Could you check a few things on this model? Use its own coordinates, in mm. A direction names the side the tool comes from. Coordinates: 2 decimals unless noted, no trailing zeros. Order: outer loops, then holes, each group sorted by start corner. A loop starts at its lowest first (then second) coordinate and runs counter-clockwise, first axis right, second up. Notation, with made-up numbers: (58, 51) - (77, 51) arc R13 cw to (77, 57) - close; hole circle Ø1 at (3, -14). An arc over 180 degrees is marked (long way). Answer as a JSON object with one key per item and string values. Group by question number.
(1) Imagine slicing it at D-D, the plane z = 5.25. Give the number of separate pieces and of enclosed holes in the cut face, and give its area (3 significant figures).
(2) Will this pin go through, and if not, where does the flat tip stop? P1, Ø0.5, axis at y = -43.5, z = 6.5, coming from the -X side.
(3) Please list where these lines run through material, in increasing order: probe 1 along Y at (x, z) = (-43.8, 2.75); probe 2 along Y at (x, z) = (-7, 4.5); probe 3 along Y at (x, z) = (43.8, 3.5).
(4) Imagine slicing it at C-C, the plane y = 24.4. Write out the boundary of the cut face in (x, z).
(5) Imagine slicing it at A-A, the plane x = -21.5. Write out the boundary of the cut face in (y, z), and give its area (3 significant figures).
(6) We'd pull the mould along X, two halves only. Please class faces 1 (the flat face through (54.3, 30, 3)), 2 (the cylindrical face through (-52.96, 46.287, 3.296)), 3 (the cylindrical face through (48.33, -43.97, 1.01)), 4 (the cylindrical face through (-48.12, 42.39, 4.75)): pulls with the +X half, pulls with the -X half, needs draft (parallel to the pull), parting line crosses it, or undercut.
(7) Imagine slicing it at B-B, the plane x = -43.8. Write out the boundary of the cut face in (y, z), and give its area (3 significant figures).
(8) Which directions (+Z, -Z, +X, -X, +Y, -Y) give clear straight access to the entire face, cutting with the end or side of a thin tool? Please do faces 5 (the cylindrical face through (-48.12, -43.61, 1.01)), 6 (the cylindrical face through (51.91, 11.77, 3.3)), 7 (the cylindrical face through (50.352, -26.595, 7.955)).
from build123d import *

# Parameters (mm, degrees)
SKETCH1_W                = 108.6
SKETCH1_H                = 95.4
BOSS_EXTRUDE1_DEPTH      = 6.5
FILLET1_R                = 4.7
CUT_EXTRUDE2_DEPTH       = 73.567416931
SHELL1_T                 = -3
SHELL1_THICKNESS_2_DEPTH = 1
SKETCH3_W                = 21
SKETCH3_H                = 9.8
CUT_EXTRUDE1_DEPTH       = 73.567416931
BOSS_EXTRUDE2_START      = 2.87
BOSS_EXTRUDE2_DEPTH      = 2.87
SKETCH6_R                = 1.6
CUT_EXTRUDE3_DEPTH       = 73.650512042
BOSS_EXTRUDE3_START      = 7.37
SKETCH7_R                = 4.5
SKETCH7_R_2              = 1.6
BOSS_EXTRUDE3_DEPTH      = 7.37


with BuildPart() as part:
    # Sketch1 → Boss-Extrude1 (new body)
    with BuildSketch(Plane.XY):
        Rectangle(SKETCH1_W, SKETCH1_H)
    extrude(amount=BOSS_EXTRUDE1_DEPTH)

    # Fillet1
    fillet1_edges = [part.edges().sort_by_distance(p)[0] for p in [
        (54.3, -47.7, 3.25),
        (-54.3, -47.7, 3.25),
        (-54.3, 47.7, 3.25),
        (54.3, 47.7, 3.25),
    ]]
    fillet(fillet1_edges, radius=FILLET1_R)

    # Sketch4 → Cut-Extrude2 (cut, through all)
    with BuildSketch(Plane.XY.offset(6.5)):
        with BuildLine():
            Line((50.037, 6.46747704), (50.037, -20.87017704))
            ThreePointArc((50.037, -20.87017704), (146.29602, -7.20135), (50.037, 6.46747704))
        make_face()
    extrude(amount=-CUT_EXTRUDE2_DEPTH, mode=Mode.SUBTRACT)

    # Shell1
    shell1_openings = [part.faces().sort_by_distance(p)[0] for p in [
        (-0.847501067, 0.116576538, 6.5),
    ]]
    offset(amount=SHELL1_T, openings=shell1_openings, kind=Kind.INTERSECTION)

    # Shell1 thickness 2 face (on inner face of the shell) → Shell1 thickness 2 (cut)
    with BuildSketch(Plane(origin=(-0.931808726, 0.135963236, 3), x_dir=(-1, 0, 0), z_dir=(0, 0, -1))):
        with BuildLine():
            ThreePointArc((50.368191274, -43.135963236), (49.870272802, -44.338044764), (48.668191274, -44.835963236))
            Line((48.668191274, -44.835963236), (-50.531808726, -44.835963236))
            ThreePointArc((-50.531808726, -44.835963236), (-51.733890254, -44.338044764), (-52.231808726, -43.135963236))
            Line((-52.231808726, -43.135963236), (-52.231808726, -31.994266579))
            ThreePointArc((-52.231808726, -31.994266579), (-49.810478696, -26.826892146), (-47.968808726, -21.425702521))
            Line((-47.968808726, -21.425702521), (-47.968808726, 6.751076049))
            ThreePointArc((-47.968808726, 6.751076049), (-49.810478696, 12.152265674), (-52.231808726, 17.319640107))
            Line((-52.231808726, 17.319640107), (-52.231808726, 42.864036764))
            ThreePointArc((-52.231808726, 42.864036764), (-51.733890254, 44.066118292), (-50.531808726, 44.564036764))
            Line((-50.531808726, 44.564036764), (48.668191274, 44.564036764))
            ThreePointArc((48.668191274, 44.564036764), (49.870272802, 44.066118292), (50.368191274, 42.864036764))
            Line((50.368191274, 42.864036764), (50.368191274, -43.135963236))
        make_face()
    extrude(amount=SHELL1_THICKNESS_2_DEPTH, mode=Mode.SUBTRACT)

    # Sketch3 → Cut-Extrude1 (cut, through all)
    with BuildSketch(Plane.XY.offset(6.5)):
        with Locations((-15.1, -31.9)):
            Rectangle(SKETCH3_W, SKETCH3_H)
        with Locations((15.3, -31.9)):
            Rectangle(SKETCH3_W, SKETCH3_H)
    extrude(amount=-CUT_EXTRUDE1_DEPTH, mode=Mode.SUBTRACT)

    # Sketch5 → Boss-Extrude2 (add)
    with BuildSketch(Plane.XY.offset(6.5).offset(BOSS_EXTRUDE2_START)):
        with BuildLine():
            Line((52.7, 17.100794024), (52.7, 43))
            ThreePointArc((52.7, 43), (51.792031022, 45.192031022), (49.6, 46.1))
            Line((49.6, 46.1), (-49.6, 46.1))
            ThreePointArc((-49.6, 46.1), (-51.792031022, 45.192031022), (-52.7, 43))
            Line((-52.7, 43), (-52.7, -43))
            ThreePointArc((-52.7, -43), (-51.792031022, -45.192031022), (-49.6, -46.1))
            Line((-49.6, -46.1), (49.6, -46.1))
            ThreePointArc((49.6, -46.1), (51.792031022, -45.192031022), (52.7, -43))
            Line((52.7, -43), (52.7, -31.503494024))
            ThreePointArc((52.7, -31.503494024), (50.322512039, -26.523985726), (48.500249857, -21.315597065))
            Line((48.500249857, -21.315597065), (47.044269983, -21.315597065))
            ThreePointArc((47.044269983, -21.315597065), (48.883695535, -26.70338335), (51.3, -31.858303343))
            Line((51.3, -31.858303343), (51.3, -43))
            ThreePointArc((51.3, -43), (50.802081528, -44.202081528), (49.6, -44.7))
            Line((49.6, -44.7), (-49.6, -44.7))
            ThreePointArc((-49.6, -44.7), (-50.802081528, -44.202081528), (-51.3, -43))
            Line((-51.3, -43), (-51.3, 43))
            ThreePointArc((-51.3, 43), (-50.802081528, 44.202081528), (-49.6, 44.7))
            Line((-49.6, 44.7), (49.6, 44.7))
            ThreePointArc((49.6, 44.7), (50.802081528, 44.202081528), (51.3, 43))
            Line((51.3, 43), (51.3, 17.455603343))
            ThreePointArc((51.3, 17.455603343), (48.883695535, 12.30068335), (47.044269983, 6.912897065))
            Line((47.044269983, 6.912897065), (48.500249857, 6.912897065))
            ThreePointArc((48.500249857, 6.912897065), (50.322512039, 12.121285726), (52.7, 17.100794024))
        make_face()
    extrude(amount=-BOSS_EXTRUDE2_DEPTH)

    # Sketch6 → Cut-Extrude3 (cut, through all)
    with BuildSketch(Plane.XY.offset(2)):
        with Locations((-49.6, 43)):
            Circle(SKETCH6_R)
        with Locations((-43.8, 24.4)):
            Circle(SKETCH6_R)
        with Locations((43.8, 24.4)):
            Circle(SKETCH6_R)
        with Locations((49.6, 43)):
            Circle(SKETCH6_R)
        with Locations((49.6, -43)):
            Circle(SKETCH6_R)
        with Locations((44.2, -40.5)):
            Circle(SKETCH6_R)
        with Locations((-49.6, -43)):
            Circle(SKETCH6_R)
        with Locations((-43.8, -40.5)):
            Circle(SKETCH6_R)
    extrude(amount=-CUT_EXTRUDE3_DEPTH, mode=Mode.SUBTRACT)

    # Sketch7 → Boss-Extrude3 (add)
    # profile 1 of 6: a face of its own
    with BuildSketch(Plane.XY.offset(2).offset(BOSS_EXTRUDE3_START)):
        with Locations(Location((-43.8, 24.4, 0), (0, 0, 180))):
            Circle(SKETCH7_R)
        with Locations((-43.8, 24.4)):
            Circle(SKETCH7_R_2, mode=Mode.SUBTRACT)
    # profile 2 of 6: a face of its own
    with BuildSketch(Plane.XY.offset(2).offset(BOSS_EXTRUDE3_START)):
        with Locations(Location((43.8, 24.4, 0), (0, 0, 180))):
            Circle(SKETCH7_R)
        with Locations((43.8, 24.4)):
            Circle(SKETCH7_R_2, mode=Mode.SUBTRACT)
    # profile 3 of 6: a face of its own
    with BuildSketch(Plane.XY.offset(2).offset(BOSS_EXTRUDE3_START)):
        with BuildLine():
            Line((47.072281323, -38.5), (51.3, -38.5))
            Line((51.3, -38.5), (51.3, -43))
            ThreePointArc((51.3, -43), (50.802081528, -44.202081528), (49.6, -44.7))
            Line((49.6, -44.7), (41.9, -44.7))
            Line((41.9, -44.7), (41.9, -43.138181192))
            ThreePointArc((41.9, -43.138181192), (41.863323371, -37.894248222), (47.072281323, -38.5))
        make_face()
        with Locations((44.2, -40.5)):
            Circle(SKETCH7_R_2, mode=Mode.SUBTRACT)
    # profile 4 of 6: a face of its own
    with BuildSketch(Plane.XY.offset(2).offset(BOSS_EXTRUDE3_START)):
        with BuildLine():
            Line((-49.6, -44.7), (-41.9, -44.7))
            Line((-41.9, -44.7), (-41.9, -43.439387691))
            ThreePointArc((-41.9, -43.439387691), (-41.282914297, -38.068070814), (-46.672281323, -38.5))
            Line((-46.672281323, -38.5), (-51.3, -38.5))
            Line((-51.3, -38.5), (-51.3, -43))
            ThreePointArc((-51.3, -43), (-50.802081528, -44.202081528), (-49.6, -44.7))
        make_face()
        with Locations((-43.8, -40.5)):
            Circle(SKETCH7_R_2, mode=Mode.SUBTRACT)
    # profile 5 of 6: a face of its own
    with BuildSketch(Plane.XY.offset(2).offset(BOSS_EXTRUDE3_START)):
        with BuildLine():
            Line((-49.6, 44.7), (-45.433466669, 44.7))
            ThreePointArc((-45.433466669, 44.7), (-46.418019485, 39.818019485), (-51.3, 38.833466669))
            Line((-51.3, 38.833466669), (-51.3, 43))
            ThreePointArc((-51.3, 43), (-50.802081528, 44.202081528), (-49.6, 44.7))
        make_face()
        with Locations((-49.6, 43)):
            Circle(SKETCH7_R_2, mode=Mode.SUBTRACT)
    # profile 6 of 6: a face of its own
    with BuildSketch(Plane.XY.offset(2).offset(BOSS_EXTRUDE3_START)):
        with BuildLine():
            Line((45.433466669, 44.7), (49.6, 44.7))
            ThreePointArc((49.6, 44.7), (50.802081528, 44.202081528), (51.3, 43))
            Line((51.3, 43), (51.3, 38.833466669))
            ThreePointArc((51.3, 38.833466669), (46.418019485, 39.818019485), (45.433466669, 44.7))
        make_face()
        with Locations((49.6, 43)):
            Circle(SKETCH7_R_2, mode=Mode.SUBTRACT)
    extrude(amount=-BOSS_EXTRUDE3_DEPTH)


solid = part.part
Result set:
{
 "1": {"separate pieces": "3", "enclosed holes": "7", "area": "1,460 mm^2"},
 "2": {"P1": "stops at x = -54.29"},
 "3": {"probe 1": "y = -47.7 to -42.1, -38.9 to -37, 19.9 to 22.8, 26 to 28.9, 44.7 to 47.7", "probe 2": "y = -47.7 to -44.7, 44.7 to 47.7", "probe 3": "y = -47.7 to -42.05, -38.95 to -37.02, 19.9 to 22.8, 26 to 28.9, 44.7 to 47.7"},
 "4": {"outline": "(-54.3, 0) - (-45.4, 0) - (-45.4, 9.37) - (-48.3, 9.37) - (-48.3, 2) - (-51.3, 2) - (-51.3, 9.37) - (-52.7, 9.37) - (-52.7, 6.5) - (-54.3, 6.5) - close; (-42.2, 0) - (42.2, 0) - (42.2, 9.37) - (39.3, 9.37) - (39.3, 2) - (-39.3, 2) - (-39.3, 9.37) - (-42.2, 9.37) - close; (45.4, 0) - (54.3, 0) - (54.3, 6.5) - (52.7, 6.5) - (52.7, 9.37) - (51.3, 9.37) - (51.3, 2) - (48.3, 2) - (48.3, 9.37) - (45.4, 9.37) - close"},
 "5": {"outline": "(-47.7, 0) - (-36.8, 0) - (-36.8, 2) - (-44.7, 2) - (-44.7, 9.37) - (-46.1, 9.37) - (-46.1, 6.5) - (-47.7, 6.5) - close; (-27, 0) - (47.7, 0) - (47.7, 6.5) - (46.1, 6.5) - (46.1, 9.37) - (44.7, 9.37) - (44.7, 2) - (-27, 2) - close", "area": "206 mm^2"},
 "6": {"face 1": "pulls with the +X half", "face 2": "pulls with the -X half", "face 3": "undercut", "face 4": "undercut"},
 "7": {"outline": "(-47.7, 0) - (-42.1, 0) - (-42.1, 9.37) - (-46.1, 9.37) - (-46.1, 6.5) - (-47.7, 6.5) - close; (-38.9, 0) - (22.8, 0) - (22.8, 9.37) - (19.9, 9.37) - (19.9, 2) - (-37, 2) - (-37, 9.37) - (-38.9, 9.37) - close; (26, 0) - (47.7, 0) - (47.7, 6.5) - (46.1, 6.5) - (46.1, 9.37) - (44.7, 9.37) - (44.7, 2) - (28.9, 2) - (28.9, 9.37) - (26, 9.37) - close", "area": "289 mm^2"},
 "8": {"face 5": "-Z", "face 6": "+Z, -Z, +X", "face 7": "+Z, +X"}
}
